For this review, use the dimensioned drawing (mm, ordinates from the lowest corner) and the shaded views. A direction names the side the tool comes from. Give positions to 0.01 mm unless a question says otherwise; leave off trailing zeros. Order: outer loops, then holes, each group sorted by start corner. A loop starts at its lowest first (then second) coordinate and runs counter-clockwise, first axis right, second up.
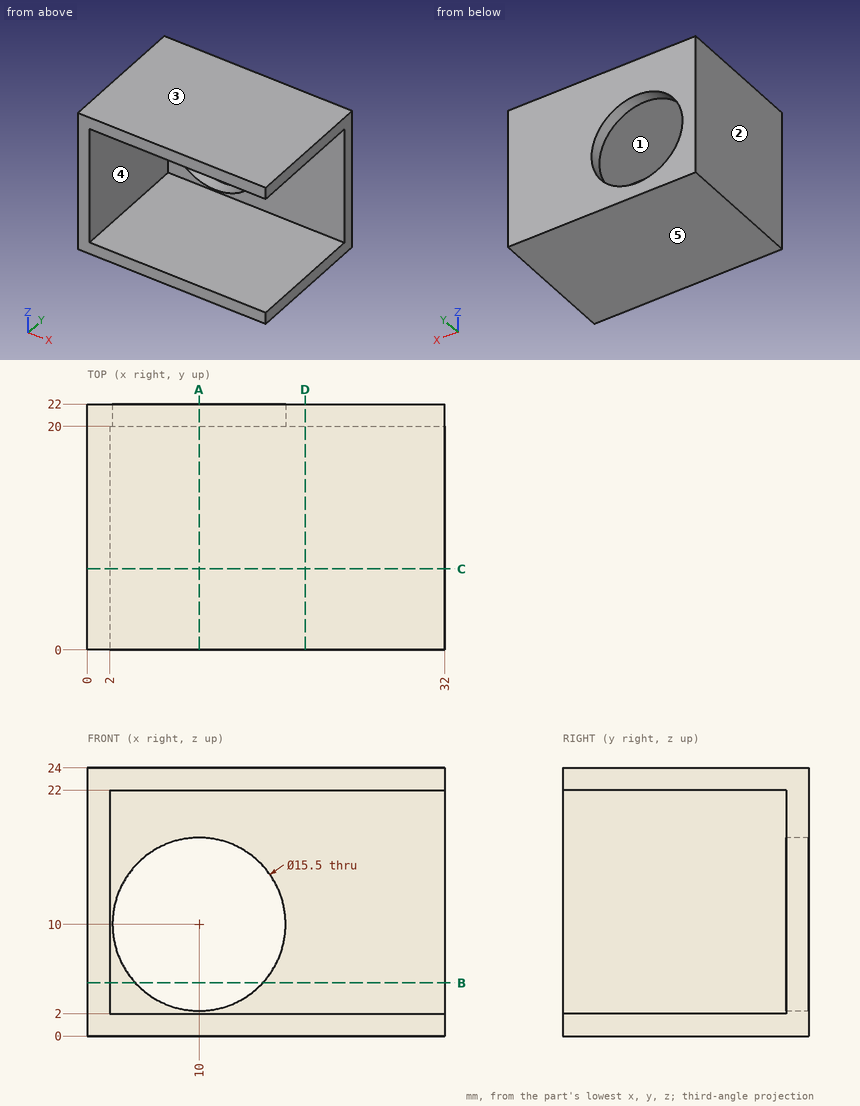
1. Take a section at D-D (x = 19.5). State the section outline as (y, z) points.
Recorded:
outline: (0, 0) - (22, 0) - (22, 24) - (0, 24) - (0, 22) - (20, 22) - (20, 2) - (0, 2) - close
2. Take a section at B-B (z = 4.75). State the section outline as (x, y) points, then the cut area to 3 significant figures.
Recorded:
outline: (0, 0) - (2, 0) - (2, 20) - (4.3, 20) - (4.3, 22) - (0, 22) - close; (15.7, 20) - (32, 20) - (32, 22) - (15.7, 22) - close
area: 81.2 mm2
3. For pin 1 (6 mm diameter, centred on y = 14.5, z = 12, fed in from +X), flat-tipped, find the tip position at first contact; note if it passes through.
Recorded:
pin 1: stops at x = 2
4. For line 1 along X through (y, z) = (20.7, 10); line 2 along Z through (x, y) = (3, 10); line 3 along Y through (x, z) = (25, 12), list the stretches that pass through material, from the lowest coordinate up.
Recorded:
line 1: x = 0 to 2.25, 17.75 to 32
line 2: z = 0 to 2, 22 to 24
line 3: y = 20 to 22
5. Take a section at A-A (x = 10). State the section outline as (y, z) points, then the cut area to 3 significant figures.
Recorded:
outline: (0, 0) - (22, 0) - (22, 2.25) - (20, 2.25) - (20, 2) - (0, 2) - close; (0, 22) - (20, 22) - (20, 17.75) - (22, 17.75) - (22, 24) - (0, 24) - close
area: 97.0 mm2
6. Take a section at C-C (y = 7.25). State the section outline as (x, z) points, then the cut area to 3 significant figures.
Recorded:
outline: (0, 0) - (32, 0) - (32, 2) - (2, 2) - (2, 22) - (32, 22) - (32, 24) - (0, 24) - close
area: 168 mm2
7. Machinability: for the marked faces 4 and 5, which of the approach directions +Z, -Z, +X, -X, +Y, -Y give a long, thin tool a straight path to every point of the face, cutting with its end or side? Answer none if there is none.
Recorded:
face 4: +X, -Y
face 5: -Z, +X, -X, +Y, -Y
8. Draft analysis for pull direction Z (two halves, no side actions). For the marked faces 1, 2 and 3, state which applies: pulls with the +Z half, pulls with the -Z half, needs draft (parallel to the pull), parting line crosses it, or undercut.
Recorded:
face 1: undercut
face 2: needs draft
face 3: pulls with the +Z half
